```python
from build123d import *

# Parameters (mm, degrees)
SKETCH_1_R                   = 40
SKETCH_1_R_2                 = 32.5
EXTRUDE_1_DEPTH              = 4
HOLE_WIZARD_M3_1_D           = 3.4
HOLE_WIZARD_M3_1_CSINK_D     = 6.72
HOLE_WIZARD_M3_1_CSINK_ANGLE = 90
EXTRUDE_START                = -4
SKETCH_4_R                   = 1.55
EXTRUDE_2_DEPTH              = 4
FILLET_1_R                   = 10
SKETCH_5_W                   = 15
SKETCH_5_H                   = 4.9
EXTRUDE_3_DEPTH              = 4


with BuildPart() as part:
    # 草图1 → 凸台-拉伸1 (new body)
    with BuildSketch(Plane.XY):
        Circle(SKETCH_1_R)
        Circle(SKETCH_1_R_2, mode=Mode.SUBTRACT)
    extrude(amount=EXTRUDE_1_DEPTH)

    # M3 六角凹锥坑螺钉的锥形沉头孔1 (through all)
    with Locations(Plane.XY.offset(4)):
        with Locations((27.960622174, 23.461747754), (36.5, 0), (27.960622174, -23.461747754), (6.338158485, -35.945482985), (-18.25, -31.609927238), (-34.298780659, -12.483735231), (-34.298780659, 12.483735231), (-18.25, 31.609927238), (6.338158485, 35.945482985)):
            CounterSinkHole(HOLE_WIZARD_M3_1_D / 2, HOLE_WIZARD_M3_1_CSINK_D / 2, counter_sink_angle=HOLE_WIZARD_M3_1_CSINK_ANGLE)

    # 草图4 → 凸台-拉伸2 (add)
    with BuildSketch(Plane.XY.offset(4).offset(EXTRUDE_START)):
        with BuildLine():
            Line((90, 57.5), (105, 57.5))
            ThreePointArc((105, 57.5), (85.710698364, 11.288182733), (39.291321381, -7.496136613))
            ThreePointArc((39.291321381, -7.496136613), (39.999999743, 0.004535468), (39.289620447, 7.505046646))
            ThreePointArc((39.289620447, 7.505046646), (75.103283481, 21.894389644), (90, 57.5))
        make_face()
        with Locations((45.011455208, 0.21880486)):
            Circle(SKETCH_4_R, mode=Mode.SUBTRACT)
        with Locations((80.658639918, 16.841360082)):
            Circle(SKETCH_4_R, mode=Mode.SUBTRACT)
        with Locations((97.28119514, 52.488544792)):
            Circle(SKETCH_4_R, mode=Mode.SUBTRACT)
        with BuildLine():
            ThreePointArc((55.681924073, -0.932245014), (65.568404835, 2.668378884), (74.681550102, 7.927426106))
            ThreePointArc((74.681550102, 7.927426106), (75.419947976, 12.105316552), (71.24205753, 12.843714426))
            ThreePointArc((71.24205753, 12.843714426), (63.032695265, 8.106225607), (54.126691933, 4.862688376))
            ThreePointArc((54.126691933, 4.862688376), (52.006841308, 1.187605611), (55.681924073, -0.932245014))
        make_face(mode=Mode.SUBTRACT)
        with BuildLine():
            ThreePointArc((89.572573894, 22.818449898), (94.831621116, 31.931595165), (98.432245014, 41.818075927))
            ThreePointArc((98.432245014, 41.818075927), (96.312394389, 45.493158692), (92.637311624, 43.373308067))
            ThreePointArc((92.637311624, 43.373308067), (89.393774393, 34.467304735), (84.656285574, 26.25794247))
            ThreePointArc((84.656285574, 26.25794247), (85.394683448, 22.080052024), (89.572573894, 22.818449898))
        make_face(mode=Mode.SUBTRACT)
    extrude(amount=EXTRUDE_2_DEPTH)

    # 圆角1
    fillet_1_edges = [part.edges().sort_by_distance(p)[0] for p in [
        (39.289620447, 7.505046646, 2),
        (39.291321381, -7.496136613, 2),
    ]]
    fillet(fillet_1_edges, radius=FILLET_1_R)

    # 草图5 → 凸台-拉伸3 (add)
    with BuildSketch(Plane.XY.offset(4)):
        with Locations((97.5, 59.95)):
            Rectangle(SKETCH_5_W, SKETCH_5_H)
    extrude(amount=-EXTRUDE_3_DEPTH)


solid = part.part
```
CAD build for the part. Positions are in the model's coordinates, mm. A direction names the side the tool comes from. Coordinates: 2 decimals unless noted, no trailing zeros. Write each loop counter-clockwise with the first axis right and the second up, starting at its lowest first coordinate (ties: lowest second). Pieces come first, ordered by that corner, then holes.
(1) Cut at D-D, the plane x = 59. List the corners of the cut face in (y, z).
(2) Flat gauge pins, fed straight in: pin 1 (1 mm diameter, centred on x = 36.5, y = 9.5, fed in from -Z); pin 2 (1.2 mm diameter, centred on y = 59, z = 1.5, fed in from -X); pin 3 (5.5 mm diameter, centred on x = -34.3, y = -12.48, fed in from +Z). Where does each tip first touch, or does it go through?
(3) Two-plate mould, pull along X, no slides. Class faces 1 (the face through (-39.983, 1.183, 1.972)), 2 (the face through (88.497, 14.221, 1.972)), 3 (the face through (32, 8, 0)): +X half, -X half, draft (parallel to the pull), parting line (faces both ways), or undercut.
(4) Cut at B-B, the plane x = -18.25. List the corners of the cut face in (y, z), and give its area (3 significant figures).
(5) 3-axis set-ups, long thin cutter, end or side, ignore diameter. For faces 4 (the face through (77.85, 24.83, 1.97)), 5 (the face through (65.435, 2.606, 1.972)): which of +Z, -Z, +X, -X, +Y, -Y reach the whole face in a straight line?
(6) Cut at C-C, the plane z = 1.6. Count the separate pieces of the cut face and the enclosed holes in it, and give its area (3 significant figures).
(7) Cut at A-A, the plane x = 0. List the corners of the cut face in (y, z), and give its area (3 significant figures).
(8) Drill centre lines: probe 1 along Y at (x, z) = (-18.25, 1.6); probe 2 along X at (y, z) = (13, 1.2); probe 3 along Y at (x, z) = (71.5, 2.95). Where is each one in solid material? Low to high.
Geometry says:
1. outline: (-4.66, 0) - (0.06, 0) - (0.06, 4) - (-4.66, 4) - close; (6.42, 0) - (11.25, 0) - (11.25, 4) - (6.42, 4) - close
2. pin 1: stops at z = 0
2. pin 2: stops at x = 90
2. pin 3: stops at z = 3.39
3. face 1: undercut
3. face 2: +X half
3. face 3: draft
4. outline: (-35.59, 0) - (-33.31, 0) - (-33.31, 2.34) - (-34.97, 4) - (-35.59, 4) - close; (-29.91, 0) - (-26.89, 0) - (-26.89, 4) - (-28.25, 4) - (-29.91, 2.34) - close; (26.89, 0) - (29.91, 0) - (29.91, 2.34) - (28.25, 4) - (26.89, 4) - close; (33.31, 0) - (35.59, 0) - (35.59, 4) - (34.97, 4) - (33.31, 2.34) - close
4. area: 36.9 mm2
5. face 4: +Z, -Z, +Y
5. face 5: +Z, -Z
6. separate pieces: 1
6. enclosed holes: 15
6. area: 2,760 mm2
7. outline: (-40, 0) - (-32.5, 0) - (-32.5, 4) - (-40, 4) - close; (32.5, 0) - (40, 0) - (40, 4) - (32.5, 4) - close
7. area: 60.0 mm2
8. probe 1: y = -35.59 to -33.31, -29.91 to -26.89, 26.89 to 29.91, 33.31 to 35.59
8. probe 2: x = -37.83 to -35.92, -32.68 to -29.79, 29.79 to 38, 62.8 to 71.49, 74.43 to 87.38
8. probe 3: y = 0.64 to 5.85, 13.01 to 18.67
